```python
from build123d import *

# Parameters (mm, degrees)
SKETCH1_R           = 12.5
BOSS_EXTRUDE1_DEPTH = 45
SKETCH2_R           = 10
BOSS_EXTRUDE2_DEPTH = 60
CHAMFER1_SIZE       = 1


with BuildPart() as part:
    # Sketch1 → Boss-Extrude1 (new body)
    with BuildSketch(Plane(origin=(0, 0, 0), x_dir=(1, 0, 0), z_dir=(0, 1, 0))):
        Circle(SKETCH1_R)
    extrude(amount=BOSS_EXTRUDE1_DEPTH)

    # Sketch2 → Boss-Extrude2 (add)
    with BuildSketch(Plane(origin=(0, 45, 0), x_dir=(1, 0, 0), z_dir=(0, 1, 0))):
        Circle(SKETCH2_R)
    extrude(amount=BOSS_EXTRUDE2_DEPTH)

    # Chamfer1
    chamfer1_edges = [part.edges().sort_by_distance(p)[0] for p in [
        (-10, 105, 0),
    ]]
    chamfer(chamfer1_edges, length=CHAMFER1_SIZE)


solid = part.part
```
Work out the finished part from the listing and answer in its coordinate system (mm). A direction names the side the tool comes from. Coordinates: 2 decimals unless noted, no trailing zeros. Loops run counter-clockwise (first coordinate to the right, second up) from the corner with the lowest first, then second, coordinate; pieces in that order, holes last. Notation, with made-up numbers: (4.5, -16) -> (9.5, -16) arc R31 cw to (9.5, 8) -> close; hole circle Ø6 at (10.25, -15.75). An arc over 180 degrees is marked (long way). Answer as CSV lines item,"result".
Q1. The part is cut by section A-A on z = 0. Write down the section's boundary in (x, y), and give its area (3 significant figures).
Findings:
outline,"(-12.5, 0) -> (12.5, 0) -> (12.5, 45) -> (10, 45) -> (10, 104) -> (9, 105) -> (-9, 105) -> (-10, 104) -> (-10, 45) -> (-12.5, 45) -> close"
area,"2,320 mm²"
Q2. Find the intervals of material crossed by probe 1 along X at (y, z) = (11, 0.5); probe 2 along Y at (x, z) = (0.25, -10.5); probe 3 along X at (y, z) = (30.5, -5.25), in increasing order.
Findings:
probe 1,"x = -12.49 to 12.49"
probe 2,"y = 0 to 45"
probe 3,"x = -11.34 to 11.34"
Q3. For a pull along Z with two mould halves and no side action, classify faces 1 (the face through (0, 0, 0)), 2 (the face through (11.923, 22.185, -3.755)) as +Z half, -Z half, draft (parallel to the pull), parting line (faces both ways), or undercut.
Findings:
face 1,"draft"
face 2,"parting line"
Q4. Each of these flat-tipped pins is pushed along its axis until it touches: pin 1 (6 mm diameter, centred on y = 88.5, z = -3.5, fed in from +X); pin 2 (3 mm diameter, centred on y = 31, z = -8, fed in from -X); pin 3 (4 mm diameter, centred on x = 3.5, y = 88, fed in from +Z). Where does it stop, or does it pass through?
Findings:
pin 1,"stops at x = 9.99"
pin 2,"stops at x = -10.68"
pin 3,"stops at z = 9.89"
Q5. The part is cut by section D-D on y = 12. Write down the section's boundary in (x, z).
Findings:
outline,"circle Ø25 at (0, 0)"
Q6. A tool of negligible diameter and unlimited length cuts with its end or side. For faces 3 (the face through (0, 105, 0)), 4 (the face through (-2.17, 74.09, 9.76)), from which of +Z, -Z, +X, -X, +Y, -Y can it reach the whole face along a straight path? Write none if from no direction.
Findings:
face 3,"+Z, -Z, +X, -X, +Y"
face 4,"+Y"
Q7. The part is cut by section B-B on x = 0. Write down the section's boundary in (y, z).
Findings:
outline,"(0, -12.5) -> (45, -12.5) -> (45, -10) -> (104, -10) -> (105, -9) -> (105, 9) -> (104, 10) -> (45, 10) -> (45, 12.5) -> (0, 12.5) -> close"
Q8. The part is cut by section C-C on y = 67. Write down the section's boundary in (x, z), and give its area (3 significant figures).
Findings:
outline,"circle Ø20 at (0, 0)"
area,"314 mm²"
